The model under review builds one solid part; all positions refer to its coordinate system, in mm. Face numbers are marked on the shaded views. A direction names the side the tool comes from. Round coordinates to 2 decimals unless told otherwise and drop trailing zeros. Order: outer loops, then holes, each group sorted by start corner. A loop starts at its lowest first (then second) coordinate and runs counter-clockwise, first axis right, second up. Notation, with made-up numbers: M 77,0.25 L 108,0.25 A22 ccw 108,11.25 Z; hole C 40.5,71 d10. An arc over 180 degrees is marked long. Answer as a JSON object with one key per item and string values. Group by question number.
1) The part is to be moulded in two halves that separate along Z. For the marked faces 1, 2, 3 and 4, say which applies: +Z half, -Z half, draft (parallel to the pull), parting line (faces both ways), or undercut.
2) Consider section B-B, the plane x = -24.5. Write out the cut boundary in (y, z), then the cut area to 3 significant figures.
3) Consider section C-C, the plane y = -12. Write out the cut boundary in (x, z).
4) Consider section A-A, the plane z = 83. Write out the cut boundary in (x, y).
5) For the marked faces 5, 6, 7, 8 and 9, list the 3-axis set-ups (+Z, -Z, +X, -X, +Y, -Y) from which the entire face can be reached by the end or side of a thin tool; tool diameter is ignored.
6) Consider section D-D, the plane z = 40. Write out the cut boundary in (x, y), then the cut area to 3 significant figures.
7) Insertion check: pin 1 Ø16 at (x, z) = (-93.5, 64) entering from +Y; pin 2 Ø3.5 at (y, z) = (9, 95) entering from -X; pin 3 Ø6.5 at (y, z) = (9, 5) entering from +X; pin 4 Ø3.5 at (y, z) = (12, 13.5) entering from -X. Each pin has a flat end and moves straight along its axis. Give the tip position at first contact, or say it passes through.
8) To check wall thickness, follow line 1 (Z direction, x = -5.5, y = 9); line 2 (Z direction, x = -1, y = 9); line 3 (Y direction, x = -17, z = 19.5). State the ranges of each line that lie inside material, in increasing order.
```python
from build123d import *

# Parameters (mm, degrees)
PAD_DEPTH       = 100
SKETCH001_R     = 2
POCKET_DEPTH    = 104.001
SKETCH002_R     = 4.5
POCKET001_DEPTH = 4
POCKET002_DEPTH = 104.001
POCKET003_DEPTH = 100.001
POCKET004_DEPTH = 42.001
CHAMFER_SIZE    = 10
POCKET005_DEPTH = 16.001


with BuildPart() as part:
    # Sketch → Pad (new body)
    with BuildSketch(Plane.XY):
        Polygon((0, 0), (-70, 0), (-84.28148, -26), (-104, -26), (-104, -6), (-84.28148, -6), (-70, 4), (-6, 4), (-6, 16), (0, 16), align=None)
    extrude(amount=PAD_DEPTH)

    # Sketch001 (on Face10 of Pad) → Pocket (cut, through all)
    with BuildSketch(Plane.YZ):
        with Locations((9, 95)):
            Circle(SKETCH001_R)
        with Locations((9, 5)):
            Circle(SKETCH001_R)
    extrude(amount=-POCKET_DEPTH, mode=Mode.SUBTRACT)

    # Sketch002 (on Face2 of Pocket) → Pocket001 (cut)
    with BuildSketch(Plane.YZ):
        with Locations((9, 95)):
            Circle(SKETCH002_R)
        with Locations((9, 5)):
            Circle(SKETCH002_R)
    extrude(amount=-POCKET001_DEPTH, mode=Mode.SUBTRACT)

    # Sketch003 (on Face10 of Pocket001) → Pocket002 (cut, through all)
    with BuildSketch(Plane(origin=(-104, 0, 0), x_dir=(0, -1, 0), z_dir=(-1, 0, 0))):
        with BuildLine():
            ThreePointArc((18.5, 90), (16, 92.5), (13.5, 90))
            Line((13.5, 90), (13.5, 50))
            ThreePointArc((13.5, 50), (16, 47.5), (18.5, 50))
            Line((18.5, 50), (18.5, 90))
        make_face()
    extrude(amount=-POCKET002_DEPTH, mode=Mode.SUBTRACT)

    # Sketch004 (on Face14 of Pocket002) → Pocket003 (cut, through all)
    with BuildSketch(Plane(origin=(-100, 0, 0), x_dir=(0, -1, 0), z_dir=(-1, 0, 0))):
        with BuildLine():
            ThreePointArc((22, 90), (16, 96), (10, 90))
            Line((10, 90), (10, 50))
            ThreePointArc((10, 50), (16, 44), (22, 50))
            Line((22, 50), (22, 90))
        make_face()
    extrude(amount=-POCKET003_DEPTH, mode=Mode.SUBTRACT)

    # Sketch005 (on Face9 of Pocket003) → Pocket004 (cut, through all)
    with BuildSketch(Plane.XZ.offset(26)):
        Polygon((-104, 0), (-104, 35), (-59.98518, 35), (-10, 0), align=None)
    extrude(amount=-POCKET004_DEPTH, mode=Mode.SUBTRACT)

    # Chamfer
    chamfer_edges = [part.edges().sort_by_distance(p)[0] for p in [
        (-94.14074, -26, 100),
        (-94.14074, -26, 35),
    ]]
    chamfer(chamfer_edges, length=CHAMFER_SIZE)

    # Sketch006 (on Face4 of Chamfer) → Pocket005 (cut, through all)
    with BuildSketch(Plane.XZ):
        with BuildLine():
            ThreePointArc((0, 35), (15, 50), (0, 65))
            Line((0, 65), (-30, 65))
            ThreePointArc((-30, 65), (-45, 50), (-30, 35))
            Line((-30, 35), (0, 35))
        make_face()
    extrude(amount=-POCKET005_DEPTH, mode=Mode.SUBTRACT)


solid = part.part
```
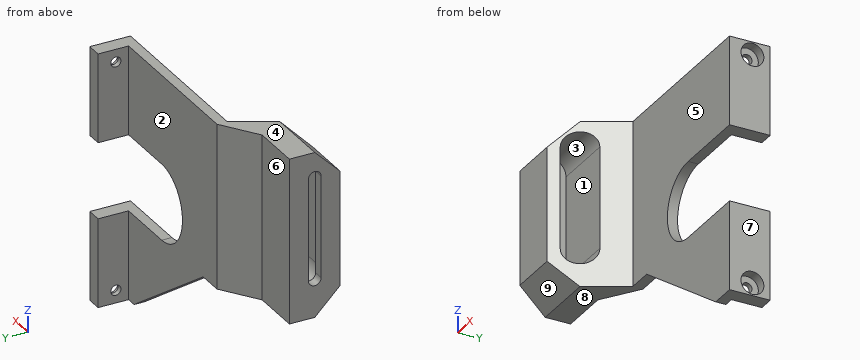
Results list:
{
 "1": {"face 1": "undercut", "face 2": "draft", "face 3": "undercut", "face 4": "+Z half"},
 "2": {"outline": "M 0,10.15 L 4,10.15 L 4,35 L 0,35 Z; M 0,65 L 4,65 L 4,100 L 0,100 Z", "area": "239 mm^2"},
 "3": {"outline": "M -104,35 L -76.59,35 L -76.59,45.53 L -100,45.53 L -100,94.47 L -76.59,94.47 L -76.59,100 L -104,100 Z"},
 "4": {"outline": "M -104,-26 L -84.28,-26 L -82.08,-22 L -100,-22 L -100,-18.5 L -104,-18.5 Z; M -104,-13.5 L -100,-13.5 L -100,-10 L -75.49,-10 L -70,0 L 0,0 L 0,16 L -6,16 L -6,4 L -70,4 L -84.28,-6 L -104,-6 Z"},
 "5": {"face 5": "+Z, -Z, +X, -Y", "face 6": "+Z, -Z, -X, +Y", "face 7": "+Z, -Z, +X, +Y, -Y", "face 8": "-Z, -X, +Y, -Y", "face 9": "-Z, +X, -X, -Y"},
 "6": {"outline": "M -104,-21 L -81.54,-21 L -70,0 L -41.18,0 L -41.18,4 L -70,4 L -84.28,-6 L -104,-6 Z", "area": "576 mm^2"},
 "7": {"pin 1": "y = -6", "pin 2": "through", "pin 3": "x = -4", "pin 4": "x = -6"},
 "8": {"line 1": "0 to 3, 7 to 35, 65 to 93, 97 to 100", "line 2": "0 to 0.5, 9.5 to 35, 65 to 90.5, 99.5 to 100", "line 3": "0 to 4"}
}
